Work out the finished part from the listing and answer in its coordinate system (mm). Round coordinates to 2 decimals unless told otherwise and drop trailing zeros. Loops run counter-clockwise (first coordinate to the right, second up) from the corner with the lowest first, then second, coordinate; pieces in that order, holes last. Notation, with made-up numbers: (48, 66) - (101, 66) arc R26 cw to (101, 88) - close; hole circle Ø8 at (41, 8.5). An arc over 180 degrees is marked (long way). Return JSON: item names as keys, results as strings.
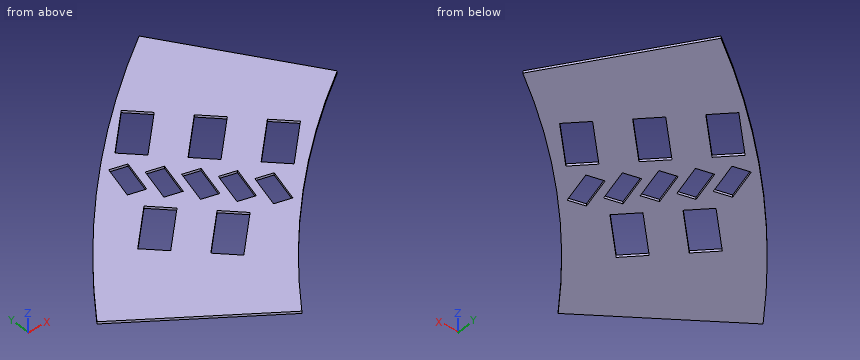
from build123d import *

# Parameters (mm, degrees)
BOSS_EXTRUDE1_DEPTH = 0.1
CUT_EXTRUDE1_DEPTH  = 102.944318085


with BuildPart() as part:
    # Sketch1 → Boss-Extrude1 (new, symmetric)
    with BuildSketch(Plane(origin=(0, 0, 0), x_dir=(0, 1, 0), z_dir=(0, 0, 1))):
        with BuildLine():
            Line((50.474726399, 72.085379897), (42.44465629, 60.617251277))
            ThreePointArc((42.44465629, 60.617251277), (52.325901808, 52.325901808), (60.617251277, 42.44465629))
            Line((60.617251277, 42.44465629), (72.085379897, 50.474726399))
            ThreePointArc((72.085379897, 50.474726399), (62.225396744, 62.225396744), (50.474726399, 72.085379897))
        make_face()
    extrude(amount=BOSS_EXTRUDE1_DEPTH, both=True)

    # Sketch2 → Cut-Extrude1 (cut, through all)
    with BuildSketch(Plane.XY.offset(0.1)):
        Polygon((-54.809835721, 52.480589816), (-54.086251462, 55.355942111), (-52.67039502, 54.999640924), (-53.393979279, 52.124288629), align=None)
        Polygon((-56.577602674, 54.248356769), (-55.854018415, 57.123709064), (-54.438161973, 56.767407877), (-55.161746232, 53.892055582), align=None)
        Polygon((-58.345369627, 56.016123722), (-57.621785368, 58.891476017), (-56.205928926, 58.53517483), (-56.929513185, 55.659822535), align=None)
        Polygon((-60.11313658, 57.783890675), (-59.389552321, 60.65924297), (-57.973695879, 60.302941783), (-58.697280138, 57.427589488), align=None)
        Polygon((-61.880903533, 59.551657628), (-61.157319274, 62.427009923), (-59.741462831, 62.070708736), (-60.465047091, 59.195356441), align=None)
        Polygon((-51.01952203, 54.862647385), (-52.617583355, 56.460708711), (-49.389640899, 59.688651167), (-47.791579573, 58.090589841), align=None)
        Polygon((-59.858356794, 49.559346526), (-56.630414338, 52.787288983), (-58.228475664, 54.385350308), (-61.45641812, 51.157407852), align=None)
        Polygon((-54.555055935, 58.398181291), (-56.153117261, 59.996242617), (-52.925174805, 63.224185073), (-51.327113479, 61.626123747), align=None)
        Polygon((-58.090589841, 61.933715197), (-59.688651167, 63.531776523), (-56.460708711, 66.759718979), (-54.862647385, 65.161657653), align=None)
        Polygon((-63.3938907, 53.094880432), (-60.165948244, 56.322822888), (-61.76400957, 57.920884214), (-64.991952026, 54.692941758), align=None)
    extrude(amount=-CUT_EXTRUDE1_DEPTH, mode=Mode.SUBTRACT)


solid = part.part
1) Section C-C (x = -55.5) is taken. Give the vertices of the cut face in (y, z).
Verdict:
{"outline": "(48.95, -0.1) - (53.98, -0.1) - (53.98, 0.1) - (48.95, 0.1) - close; (57.03, -0.1) - (59.34, -0.1) - (59.34, 0.1) - (57.03, 0.1) - close; (60.65, -0.1) - (64.52, -0.1) - (64.52, 0.1) - (60.65, 0.1) - close; (65.8, -0.1) - (68.29, -0.1) - (68.29, 0.1) - (65.8, 0.1) - close"}
2) Find the intervals of material crossed by L1, parallel to X at y = 53.5, z = 0.05; L2, parallel to X at y = 58.25, z = 0; L3, parallel to Y at x = -62.5, z = 0, in increasing order.
Verdict:
{"L1": "x = -69.87 to -63.8, -62.99 to -59.11, -57.34 to -54.55, -53.05 to -51.12", "L2": "x = -65.96 to -60, -58.49 to -57.78, -56.28 to -50.83, -47.95 to -45.64", "L3": "y = 43.76 to 53.99, 57.18 to 61.95"}
3) Section A-A (x = -49) is taken. Give the vertices of the cut face in (y, z).
Verdict:
{"outline": "(55.45, -0.1) - (56.88, -0.1) - (56.88, 0.1) - (55.45, 0.1) - close; (59.3, -0.1) - (69.98, -0.1) - (69.98, 0.1) - (59.3, 0.1) - close"}
4) Section B-B (y = 65.5) is taken. Give the vertices of the cut face in (x, z).
Verdict:
{"outline": "(-58.77, -0.1) - (-57.72, -0.1) - (-57.72, 0.1) - (-58.77, 0.1) - close; (-55.2, -0.1) - (-45.86, -0.1) - (-45.86, 0.1) - (-55.2, 0.1) - close"}
5) Section D-D (z = 0.05) is taken. Count the separate pieces of the cut face and the enclosed holes in it, and give its area (3 significant figures).
Verdict:
{"separate pieces": "1", "enclosed holes": "10", "area": "323 mm2"}
